Here's how the part is built. I have some questions about the finished solid (model axes, mm). Face numbers are marked on the shaded views. A direction names the side the tool comes from. Round coordinates to 2 decimals unless told otherwise and drop trailing zeros. Order: outer loops, then holes, each group sorted by start corner. A loop starts at its lowest first (then second) coordinate and runs counter-clockwise, first axis right, second up. Notation, with made-up numbers: (-8.75, 29) - (37.25, 29) arc R26 ccw to (37.25, 47) - close; hole circle Ø5 at (-38.75, 84). An arc over 180 degrees is marked (long way). Answer as a JSON object with one key per item and string values.
```python
from build123d import *

# Parameters (mm, degrees)
SKETCH1_W           = 26
SKETCH1_H           = 25.5
BOSS_EXTRUDE1_DEPTH = 9.463
SKETCH2_W           = 26
SKETCH2_H           = 2
BOSS_EXTRUDE3_DEPTH = 1
SKETCH3_W           = 26
SKETCH3_H           = 2
BOSS_EXTRUDE4_DEPTH = 1
CHAMFER2_SIZE       = 9.463
CHAMFER2_SIZE_2     = 25.99937882
BOSS_EXTRUDE5_DEPTH = 2
SKETCH5_W           = 9
SKETCH5_H           = 2
BOSS_EXTRUDE6_DEPTH = 40


with BuildPart() as part:
    # Sketch1 → Boss-Extrude1 (new body)
    with BuildSketch(Plane(origin=(0, 0, 0), x_dir=(1, 0, 0), z_dir=(0, 1, 0))):
        Rectangle(SKETCH1_W, SKETCH1_H)
    extrude(amount=BOSS_EXTRUDE1_DEPTH)

    # Sketch2 → Boss-Extrude3 (add)
    with BuildSketch(Plane.XY.offset(12.75)):
        with Locations((0, 3)):
            Rectangle(SKETCH2_W, SKETCH2_H)
    extrude(amount=BOSS_EXTRUDE3_DEPTH)

    # Sketch3 → Boss-Extrude4 (add)
    with BuildSketch(Plane(origin=(0, 0, -12.75), x_dir=(-1, 0, 0), z_dir=(0, 0, -1))):
        with Locations((0, 3)):
            Rectangle(SKETCH3_W, SKETCH3_H)
    extrude(amount=BOSS_EXTRUDE4_DEPTH)

    # Chamfer2
    # the kernel refuses this chamfer: 25.99937882, 9.463 mm, written as the material it takes off along each edge
    with BuildSketch(Plane(origin=(-13, 9.463, -80.197451585), x_dir=(-0.09904090225205063, -0.9950833631817486, 0), z_dir=(0, 0, 1))) as chamfer2_piece_1:
        Polygon((CHAMFER2_SIZE * 0.995083363182, CHAMFER2_SIZE * 0.0990409022521), (-CHAMFER2_SIZE_2 * 0.0990409022532, CHAMFER2_SIZE_2 * 0.995083363193), (0, 0), align=None)
    extrude(amount=160.39490317, mode=Mode.SUBTRACT)

    # Sketch4 → Boss-Extrude5 (add)
    with BuildSketch(Plane(origin=(13, 0, 0), x_dir=(0, 0, -1), z_dir=(1, 0, 0))):
        Polygon((-12.75, 0), (12.75, 0), (12.75, 2), (13.75, 2), (13.75, 4), (12.75, 4), (12.75, 9.463), (-12.75, 9.463), (-12.75, 4), (-13.75, 4), (-13.75, 2), (-12.75, 2), align=None)
    extrude(amount=BOSS_EXTRUDE5_DEPTH)

    # Sketch5 → Boss-Extrude6 (add)
    with BuildSketch(Plane(origin=(15, 0, 0), x_dir=(0, 0, -1), z_dir=(1, 0, 0))):
        with Locations((-4.5, 1)):
            Rectangle(SKETCH5_W, SKETCH5_H)
    extrude(amount=BOSS_EXTRUDE6_DEPTH)


solid = part.part
```
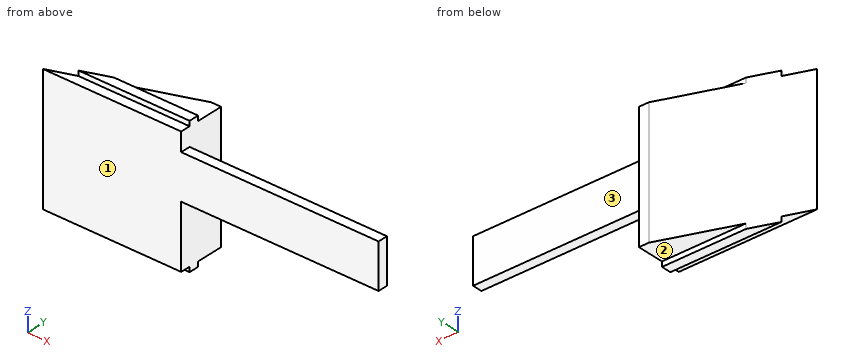
1. Imagine slicing it at D-D (z = -8.25). List the corners of the cut face in (x, y) for me.
Responses:
{"outline": "(-13, 0) - (15, 0) - (15, 9.46) - (13, 9.46) - close"}
2. Imagine slicing it at C-C (z = 6.25). List the corners of the cut face in (x, y) for me.
Responses:
{"outline": "(-13, 0) - (55, 0) - (55, 2) - (15, 2) - (15, 9.46) - (13, 9.46) - close"}
3. If I drill on L1, parallel to Z at x = -4.5, y = 1.5; L2, parallel to Z at x = 34, y = 0.5; L3, parallel to Y at x = 20, z = 8.25, over which ranges is the centre line in solid material (lowest first)? Write a range as [from, to].
Responses:
{"L1": "[-12.75, 12.75]", "L2": "[0, 9]", "L3": "[0, 2]"}
4. For the marked faces 1, 2 and 3, which set-ups out of +Z, -Z, +X, -X, +Y, -Y let a thin tool reach every point of the face, with its end or its side?
Responses:
{"face 1": "+Z, -Z, +X, -X, -Y", "face 2": "-Z, +X, -X, +Y", "face 3": "+Z, -Z, +X, +Y"}
5. Imagine slicing it at B-B (y = 1). List the corners of the cut face in (x, z) for me.
Responses:
{"outline": "(-10.25, -12.75) - (15, -12.75) - (15, 0) - (55, 0) - (55, 9) - (15, 9) - (15, 12.75) - (-10.25, 12.75) - close"}
6. Imagine slicing it at A-A (x = 3). List the corners of the cut face in (y, z) for me.
Responses:
{"outline": "(0, -12.75) - (2, -12.75) - (2, -13.75) - (4, -13.75) - (4, -12.75) - (5.82, -12.75) - (5.82, 12.75) - (4, 12.75) - (4, 13.75) - (2, 13.75) - (2, 12.75) - (0, 12.75) - close"}
7. For P1, Ø4.5, axis at x = 26.5, z = 5.5, coming from the +Y side; P2, Ø1.6, axis at x = 3.5, y = 7.5, coming from the +Z side; P3, Ø1, axis at x = 7.5, y = 0.5, coming from the +Z side; P4, Ø1.6, axis at x = 32.5, y = 1.5, coming from the -Z side, each with a flat end and sliding along its axis, tell me the tip position at first contact or that it passes through.
Responses:
{"P1": "y = 2", "P2": "through", "P3": "z = 12.75", "P4": "z = 0"}
